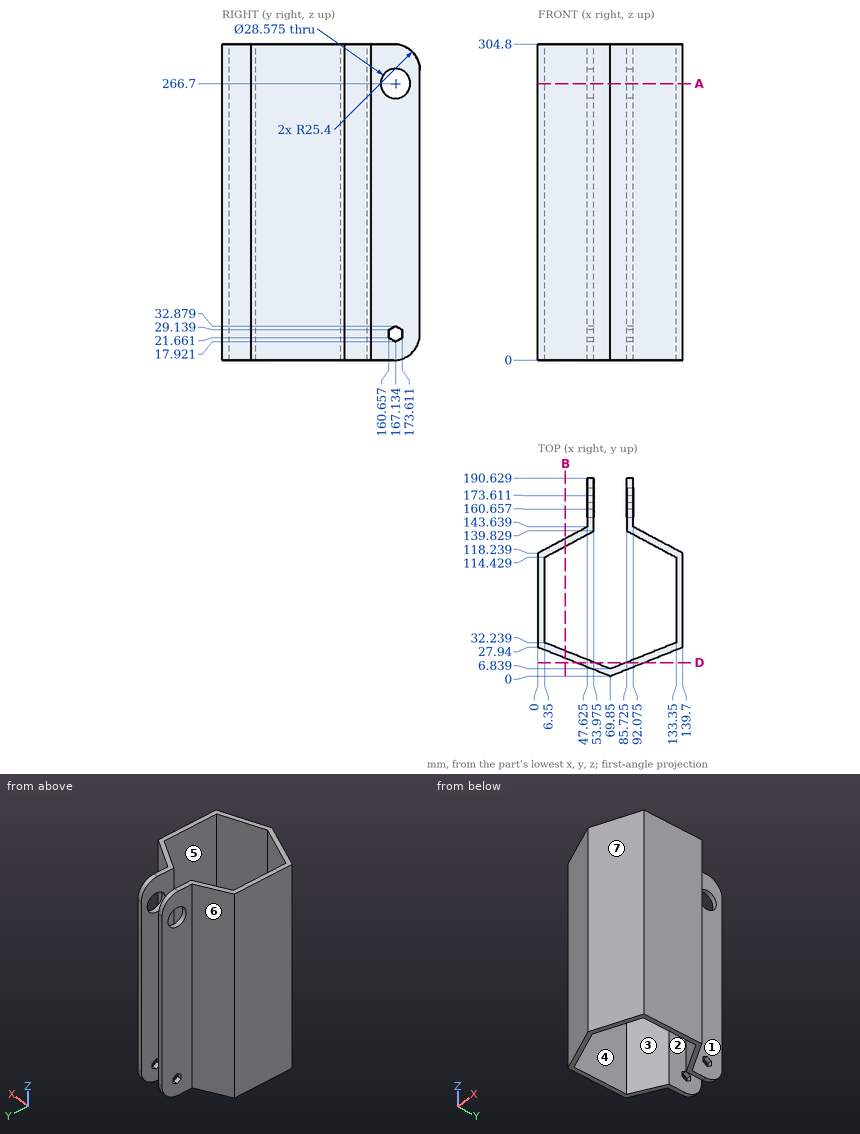
Here's the drawing with two shaded views (mm, measured from the low corner). I have some questions. A direction names the side the tool comes from. Coordinates: 2 decimals unless noted, no trailing zeros. Order: outer loops, then holes, each group sorted by start corner. A loop starts at its lowest first (then second) coordinate and runs counter-clockwise, first axis right, second up.
Item 1: If we mould it in two halves opening along X, with no side actions, what happens to the marked faces 4, 5, 6 and 7? For each: +X half, -X half, draft (parallel to the pull), parting line (faces both ways), or undercut.
Result sheet:
face 4: undercut
face 5: undercut
face 6: -X half
face 7: +X half
Item 2: If we section it at D-D on y = 13: List the corners of the cut face in (x, z) for me.
Result sheet:
outline: (37.35, 0) - (54.45, 0) - (54.45, 304.8) - (37.35, 304.8) - close; (85.25, 0) - (102.35, 0) - (102.35, 304.8) - (85.25, 304.8) - close
Item 3: I need wall thicknesses on line 1 (X direction, y = 165, z = 116.5) (1 decimal); line 2 (Y direction, x = 49.5, z = 266.7) (1 decimal); line 3 (X direction, y = 42.5, z = 167). Which ranges of each line are inside material? Lowest first, please.
Result sheet:
line 1: x = 47.6 to 54, 85.7 to 92.1
line 2: y = 8.1 to 15, 137.4 to 152.8, 181.4 to 190.6
line 3: x = 0 to 6.35, 133.35 to 139.7
Item 4: For the marked faces 1, 2 and 3, which set-ups out of +Z, -Z, +X, -X, +Y, -Y let a thin tool reach every point of the face, with its end or its side?
Result sheet:
face 1: +Z, -Z, +X, +Y
face 2: +Z, -Z, +Y
face 3: +Z, -Z
Item 5: If we section it at B-B on x = 26.5: List the corners of the cut face in (y, z) for me (1 decimal), plus the area to 3 significant figures.
Result sheet:
outline: (17.3, 0) - (24.2, 0) - (24.2, 304.8) - (17.3, 304.8) - close; (125.2, 0) - (132.4, 0) - (132.4, 304.8) - (125.2, 304.8) - close
area: 4,280 mm2
Item 6: If we section it at A-A on z = 266.7: State how many separate pieces and enclosed holes the cut face has, plus the area to 3 significant figures.
Result sheet:
separate pieces: 3
enclosed holes: 0
area: 2,950 mm2
Item 7: For P1, Ø4, axis at x = 79, z = 46.5, coming from the +Y side; P2, Ø8, axis at x = 33.5, z = 189.5, coming from the +Y side; P3, Ø5, axis at x = 28.5, z = 156, coming from the +Y side; P4, Ø24.5, axis at y = 85.5, z = 101.5, coming from the -X side, each with a flat end and sliding along its axis, tell me the tip position at first contact or that it passes through.
Result sheet:
P1: stops at y = 11.3
P2: stops at y = 138.24
P3: stops at y = 134.77
P4: stops at x = 0
